For this review, take the finished solid that the model builds, in its own axes (mm). Face numbers are marked on the shaded views. Coordinates: 2 decimals unless noted, no trailing zeros. Loops run counter-clockwise (first coordinate to the right, second up) from the corner with the lowest first, then second, coordinate; pieces in that order, holes last. Notation, with made-up numbers: (78.25, 68) - (106.25, 68) arc R21 ccw to (106.25, 94) - close; hole circle Ø6 at (83.25, 62.25). An arc over 180 degrees is marked (long way). One line per item, written item: value. Start each with the question number.
1. Insertion check: pin 1 (6 mm diameter, centred on x = -4, y = -34.5, fed in from +Z); pin 2 (1 mm diameter, centred on x = 27.5, z = 5.5, fed in from -Y). Each pin has a flat end and moves straight along its axis. Give the tip position at first contact, or say it passes through.
2. Take a section at B-B, the plane y = -3. State the section outline as (x, z) points, and give its area (3 significant figures).
3. Take a section at D-D, the plane x = 39.5. State the section outline as (y, z) points, and give its area (3 significant figures).
4. Take a section at C-C, the plane x = 58.5. State the section outline as (y, z) points, and give its area (3 significant figures).
5. To check wall thickness, follow line 1 (Z direction, x = -6, y = -33.5); line 2 (X direction, y = -2, z = 2.75); line 3 (X direction, y = -26.5, z = 6). State the ranges of each line that lie inside material, in increasing order. Write a range as from..to.
6. The part is to be moulded in two halves that separate along Y. For the marked faces 1, 2 and 3, say which applies: released by +Y, released by -Y, zero draft, split by the parting line, or undercut.
7. Take a section at A-A, the plane z = 5. State the section outline as (x, y) points, and give its area (3 significant figures).
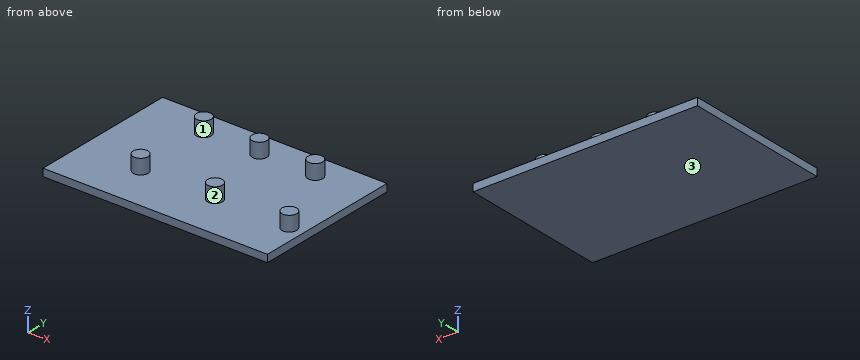
Autodesk Inventor part; units mm, degrees
ref_plane "YZ Plane" through (0, 0, 0) normal (1, 0, 0) x (0, 1, 0)
ref_plane "XZ Plane" through (0, 0, 0) normal (0, 1, 0) x (-1, 0, 0)
ref_plane "XY Plane" through (0, 0, 0) normal (0, 0, 1) x (1, 0, 0)
sketch "Sketch1" plane through (0, 0, 0) normal (0, 0, 1) x (1, 0, 0)
  line L0 (-14.3848, 7.3422) -> (87.2152, 7.3422)
  line L1 (87.2152, 7.3422) -> (87.2152, -43.4578)
  line L2 (87.2152, -43.4578) -> (-14.3848, -43.4578)
  line L3 (-14.3848, -43.4578) -> (-14.3848, 7.3422)
  point P0 (0, 0)
  dimension "d0" = 101.6
  dimension "d1" = 50.8
extrude "Extrusion1" add sketch "Sketch1" along normal blind 2.54
sketch "Sketch2" plane through (0, 0, 2.54) normal (0, 0, 1) x (1, 0, 0)
  circle A0 centre (6.7139, -1.3468) radius 2.54
  line L0 (6.7139, -1.3468) -> (25.7639, -1.3468) construction
  circle A1 centre (25.7639, -1.3468) radius 2.54
  line L1 (25.7639, -1.3468) -> (44.8139, -1.3468) construction
  circle A2 centre (44.8139, -1.3468) radius 2.54
  line L2 (-14.3848, 7.3422) -> (-14.3848, -43.4578)
  line L3 (-14.3848, -18.0578) -> (87.2152, -18.0578) construction
  line L4 (87.2152, -43.4578) -> (87.2152, 7.3422)
  circle A3 centre (6.7139, -28.1707) radius 2.54
  line L5 (6.7139, -28.1707) -> (32.1139, -28.1707) construction
  circle A4 centre (32.1139, -28.1707) radius 2.54
  line L6 (32.1139, -28.1707) -> (57.5139, -28.1707) construction
  circle A5 centre (57.5139, -28.1707) radius 2.54
  point P0 (0, 0)
  dimension "d4" = 5.08
  dimension "d5" = 19.05
  dimension "d6" = 5.08
  dimension "d7" = 19.05
  dimension "d8" = 5.08
  dimension "d9" = 5.08
  dimension "d10" = 25.4
  dimension "d11" = 5.08
  dimension "d12" = 25.4
  dimension "d13" = 5.08
extrude "Extrusion2" add sketch "Sketch2" along normal blind 5.08
sketch "Sketch3" plane through (0, 0, 2.54) normal (0, 0, 1) x (1, 0, 0)
  line L0 (87.2152, -43.4578) -> (87.2152, 7.3422)
  line L1 (-14.3848, -43.4578) -> (87.2152, -43.4578)
  line L2 (87.2152, 7.3422) -> (62.3485, 7.3422)
  line L3 (62.3485, 7.3422) -> (62.3485, -43.4578)
  line L4 (62.3485, -43.4578) -> (87.2152, -43.4578)
  line L5 (87.2152, -43.4578) -> (87.2152, 7.3422)
  point P0 (0, 0)
extrude "Extrusion3" cut sketch "Sketch3" against normal blind 5.08
properties part number "Backdrop base"
Solutions:
1. pin 1: z = 2.54
1. pin 2: y = -3.57
2. outline: (-14.38, 0) - (62.35, 0) - (62.35, 2.54) - (46.74, 2.54) - (46.74, 7.62) - (42.89, 7.62) - (42.89, 2.54) - (27.69, 2.54) - (27.69, 7.62) - (23.84, 7.62) - (23.84, 2.54) - (8.64, 2.54) - (8.64, 7.62) - (4.79, 7.62) - (4.79, 2.54) - (-14.38, 2.54) - close
2. area: 254 mm2
3. outline: (-43.46, 0) - (7.34, 0) - (7.34, 2.54) - (-43.46, 2.54) - close
3. area: 129 mm2
4. outline: (-43.46, 0) - (7.34, 0) - (7.34, 2.54) - (-25.83, 2.54) - (-25.83, 7.62) - (-30.51, 7.62) - (-30.51, 2.54) - (-43.46, 2.54) - close
4. area: 153 mm2
5. line 1: 0..2.54
5. line 2: 4.26..9.17, 23.31..28.22, 42.36..47.27
5. line 3: 4.8..8.63, 30.2..34.03, 55.6..59.43
6. face 1: undercut
6. face 2: split by the parting line
6. face 3: zero draft
7. outline: circle Ø5.08 at (6.71, -28.17); circle Ø5.08 at (6.71, -1.35); circle Ø5.08 at (25.76, -1.35); circle Ø5.08 at (32.11, -28.17); circle Ø5.08 at (44.81, -1.35); circle Ø5.08 at (57.51, -28.17)
7. area: 122 mm2
